from build123d import *

# Parameters (mm, degrees)
SKETCH1_R           = 10
SKETCH1_R_2         = 7.5
BOSS_EXTRUDE1_DEPTH = 5
BOSS_EXTRUDE2_START = 1
SKETCH1_3_R         = 10
SKETCH1_3_R_2       = 7.5
SKETCH1_3_R_3       = 4.5
BOSS_EXTRUDE2_DEPTH = 1
SKETCH2_R           = 10
BOSS_EXTRUDE3_DEPTH = 6
BOSS_EXTRUDE7_REACH = 67.17
SKETCH3_W           = 15
SKETCH3_H           = 14
SKETCH4_R           = 2
CUT_EXTRUDE4_DEPTH  = 68.699039875
CUT_EXTRUDE5_START  = 3
SKETCH4_3_R         = 2
CUT_EXTRUDE5_DEPTH  = 65.699039875
BOSS_EXTRUDE8_REACH = 69.699
CUT_EXTRUDE6_DEPTH  = 69.867191027


with BuildPart() as part:
    # Sketch1 → Boss-Extrude1 (new body)
    with BuildSketch(Plane.XY):
        Circle(SKETCH1_R)
        Circle(SKETCH1_R_2, mode=Mode.SUBTRACT)
    extrude(amount=-BOSS_EXTRUDE1_DEPTH)

    # Sketch1<3> → Boss-Extrude2 (add)
    # profile 1 of 2: a face of its own
    with BuildSketch(Plane.XY.offset(BOSS_EXTRUDE2_START)):
        Circle(SKETCH1_3_R)
        Circle(SKETCH1_3_R_2, mode=Mode.SUBTRACT)
    # profile 2 of 2: a face of its own
    with BuildSketch(Plane.XY.offset(BOSS_EXTRUDE2_START)):
        Circle(SKETCH1_3_R_2)
        Circle(SKETCH1_3_R_3, mode=Mode.SUBTRACT)
    extrude(amount=-BOSS_EXTRUDE2_DEPTH)

    # Sketch2 → Boss-Extrude3 (add)
    with BuildSketch(Plane.XY.offset(1)):
        Polygon((55, 17.6), (55, 22.6), (40, 22.6), (40, 36.3), (-12, 12.052001776), (-12, -12), (12, -12), (12, -2.451229301), align=None)
        Circle(SKETCH2_R, mode=Mode.SUBTRACT)
    extrude(amount=-BOSS_EXTRUDE3_DEPTH)

    # Boss-Extrude7: up to this plane
    boss_extrude7_end = Plane(origin=(3.082149634, -6.609691221, -87.594733488), z_dir=(-0.42261826174069755, 0.9063077870366509, 0))
    # Sketch3 → Boss-Extrude7 (add, up to the surface)
    with BuildSketch(Plane.XZ.offset(-22.6), mode=Mode.PRIVATE) as boss_extrude7_sk1:
        Polygon((40, -5), (40, -19), (10.620255189, -5), align=None)
    boss_extrude7_tool1 = split(extrude(boss_extrude7_sk1.sketch, amount=BOSS_EXTRUDE7_REACH, mode=Mode.PRIVATE), bisect_by=boss_extrude7_end, keep=Keep.BOTH, mode=Mode.PRIVATE)
    add(boss_extrude7_tool1.solids().sort_by_distance((30.206752, 22.6, -9.666667))[0])
    # Sketch3 → Boss-Extrude7 (add, up to the surface)
    with BuildSketch(Plane.XZ.offset(-22.6), mode=Mode.PRIVATE) as boss_extrude7_sk2:
        with Locations((47.5, -12)):
            Rectangle(SKETCH3_W, SKETCH3_H)
    boss_extrude7_tool2 = split(extrude(boss_extrude7_sk2.sketch, amount=BOSS_EXTRUDE7_REACH, mode=Mode.PRIVATE), bisect_by=boss_extrude7_end, keep=Keep.BOTH, mode=Mode.PRIVATE)
    add(boss_extrude7_tool2.solids().sort_by_distance((47.5, 22.6, -12))[0])

    # Sketch4 → Cut-Extrude4 (cut, through all)
    with BuildSketch(Plane.XZ.offset(-22.6)):
        with Locations((47.5, -14)):
            Circle(SKETCH4_R)
        with Locations((47.5, -4)):
            Circle(SKETCH4_R)
    extrude(amount=CUT_EXTRUDE4_DEPTH, mode=Mode.SUBTRACT)

    # Sketch4<3> → Cut-Extrude5 (cut, through all)
    # profile 1 of 2: a face of its own
    with BuildSketch(Plane.XZ.offset(-22.6).offset(CUT_EXTRUDE5_START)):
        Polygon((47.5, -8.041451884), (44, -6.020725942), (44, -1.979274058), (47.5, 0.041451884), (51, -1.979274058), (51, -6.020725942), align=None)
        with Locations(Location((47.5, -4, 0), (0, 0, 90))):
            Circle(SKETCH4_3_R, mode=Mode.SUBTRACT)
    # profile 2 of 2: a face of its own
    with BuildSketch(Plane.XZ.offset(-22.6).offset(CUT_EXTRUDE5_START)):
        Polygon((51, -16.020725942), (51, -11.979274058), (47.5, -9.958548116), (44, -11.979274058), (44, -16.020725942), (47.5, -18.041451884), align=None)
        with Locations(Location((47.5, -14, 0), (0, 0, 90))):
            Circle(SKETCH4_3_R, mode=Mode.SUBTRACT)
    extrude(amount=CUT_EXTRUDE5_DEPTH, mode=Mode.SUBTRACT)

    # Boss-Extrude8: up to this face of the body (flat: up to its plane)
    boss_extrude8_end = Plane(part.part.faces().sort_by_distance((14, 24.176000888, -2))[0])
    # Sketch3<4> → Boss-Extrude8 (add, up to the picked face)
    with BuildSketch(Plane.XZ.offset(-22.6), mode=Mode.PRIVATE) as boss_extrude8_sk1:
        Polygon((40, -5), (40, -19), (10.620255189, -5), align=None)
    boss_extrude8_tool1 = split(extrude(boss_extrude8_sk1.sketch, amount=-BOSS_EXTRUDE8_REACH, mode=Mode.PRIVATE), bisect_by=boss_extrude8_end, keep=Keep.BOTH, mode=Mode.PRIVATE)
    add(boss_extrude8_tool1.solids().sort_by(Axis((30.206752, 22.6, -9.666667), (0, 1, 0)))[0])

    # Sketch6 → Cut-Extrude6 (cut, through all)
    with BuildSketch(Plane.XY.offset(1)):
        Polygon((-12, 12.052001776), (18.725283831, 20.703901024), (15.930931538, 25.076409051), align=None)
        Polygon((15.930931538, 25.076409051), (18.725283831, 20.703901024), (40, 34.3), (40, 36.3), align=None)
    extrude(amount=-CUT_EXTRUDE6_DEPTH, mode=Mode.SUBTRACT)


solid = part.part
Geometry check sheet. Reference: the model listing, model coordinates, mm. A direction names the side the tool comes from. Give positions to 0.01 mm unless a question says otherwise; leave off trailing zeros. Order: outer loops, then holes, each group sorted by start corner. A loop starts at its lowest first (then second) coordinate and runs counter-clockwise, first axis right, second up.
1. Access from +Z, -Z, +X, -X, +Y, -Y to the whole of each face (thin tool, end or side, straight path). Record for faces 4 (the face through (45.774, 16.085, -7.045)), 5 (the face through (-7.493, 0.33, -2.465)), 6 (the face through (40, 28, -9)).
Completed:
face 4: -Y
face 5: -Z
face 6: +Z, -Z, +X, +Y
2. Depth check by flat-ended pin: pin 1 (4.5 mm diameter, centred on y = 15, z = -14.5, fed in from +X); pin 2 (6 mm diameter, centred on x = 27, y = 26, fed in from -Z); pin 3 (10 mm diameter, centred on x = 11, y = 19, fed in from -Z). Enter the tip coordinate at first touch or a pass-through.
Completed:
pin 1: stops at x = 54.25
pin 2: stops at z = -14.23
pin 3: stops at z = -7.56
3. Sectioned sample at B-B (y = 0). Record the boundary of the cut face in (x, z).
Completed:
outline: (-12, -5) - (-7.5, -5) - (-7.5, 0) - (-4.5, 0) - (-4.5, 1) - (-12, 1) - close; (4.5, 0) - (7.5, 0) - (7.5, -5) - (10.62, -5) - (17.26, -8.16) - (17.26, 1) - (4.5, 1) - close
4. Scan lines: line 1 (Z direction, x = 47.5, y = 20.3); line 2 (Z direction, x = 46, y = 18.5); line 3 (Z direction, x = -6, y = -1). Record each from-to range of solid material in increasing order.
Completed:
line 1: z = -19 to -16, -12 to -6, -2 to 1
line 2: z = -19 to -17.18, -10.82 to -7.18, -0.82 to 1
line 3: z = 0 to 1
5. Sectioned sample at C-C (x = -3.5). Record the boundary of the cut face in (y, z), then the cut area to 3 significant figures.
Completed:
outline: (-12, -5) - (-6.63, -5) - (-6.63, 0) - (-2.83, 0) - (-2.83, 1) - (-12, 1) - close; (2.83, 0) - (6.63, 0) - (6.63, -5) - (14.45, -5) - (14.45, 1) - (2.83, 1) - close
area: 86.7 mm2
6. Draft check along Y on faces 1 (the face through (-0.59, 4.46, 0.51)), 2 (the face through (49, 19.6, -6)), 3 (the face through (45.7, 16.1, -1)). Enter one of: pulls with the +Y half, pulls with the -Y half, needs draft (parallel to the pull), parting line crosses it, or undercut.
Completed:
face 1: undercut
face 2: pulls with the -Y half
face 3: needs draft
7. Sectioned sample at A-A (z = -4). Record the boundary of the cut face in (x, y).
Completed:
outline: (-12, -12) - (12, -12) - (12, -2.45) - (44, 12.47) - (44, 19.6) - (45.5, 19.6) - (45.5, 22.6) - (40, 22.6) - (40, 34.3) - (18.73, 20.7) - (-12, 12.05) - close; (49.5, 19.6) - (51, 19.6) - (51, 15.73) - (55, 17.6) - (55, 22.6) - (49.5, 22.6) - close; hole circle Ø15 at (0, 0)
8. Sectioned sample at D-D (z = -14). Record the boundary of the cut face in (x, y), then the cut area to 3 significant figures.
Completed:
outline: (29.51, 5.71) - (44, 12.47) - (44, 19.6) - (45.5, 19.6) - (45.5, 22.6) - (40, 22.6) - (40, 34.3) - (29.51, 27.59) - close; (49.5, 19.6) - (51, 19.6) - (51, 15.73) - (55, 17.6) - (55, 22.6) - (49.5, 22.6) - close
area: 316 mm2
